from build123d import *

# Parameters (mm, degrees)
F0_W           = 101.6
F0_H           = 50.8
F1_DEPTH       = 50.8
F3_D           = 12.7
F3_CBORE_D     = 25.4
F3_CBORE_DEPTH = 6.35
F5_R           = 12.7
F6_DEPTH       = 25.4
F7_R           = 5.08


with BuildPart() as f1:
    # F0 (on Top) → F1 (new body)
    with BuildSketch(Plane.XY):
        with Locations((50.8, 25.4)):
            Rectangle(F0_W, F0_H)
    extrude(amount=F1_DEPTH)

    # F3 (through all)
    with Locations(Plane(origin=(0, 50.8, 0), x_dir=(-1, 0, 0), z_dir=(0, 1, 0))):
        with Locations((-50.8, 25.4)):
            CounterBoreHole(F3_D / 2, F3_CBORE_D / 2, F3_CBORE_DEPTH)

    # F5 (on offset) → F6 (join, through all)
    with BuildSketch(Plane(origin=(0, 0, -25.4), x_dir=(1, 0, 0), z_dir=(0, 0, -1))):
        with Locations((50.8, -26.0627344251)):
            Circle(F5_R)
    extrude(amount=-F6_DEPTH)

    # F7
    f7_edges = [f1.edges().sort_by_distance(p)[0] for p in [
        (101.6, 0, 25.4),
        (101.6, 50.8, 25.4),
        (101.6, 25.4, 0),
        (101.6, 25.4, 50.8),
        (0, 50.8, 25.4),
        (0, 0, 25.4),
        (0, 25.4, 0),
        (0, 25.4, 50.8),
        (50.8, 0, 50.8),
        (50.8, 50.8, 50.8),
        (50.8, 0, 0),
        (57.15, 0, 25.4),
        (50.8, 50.8, 0),
    ]]
    fillet(f7_edges, radius=F7_R)


solid = f1.part
For this review, take the finished solid that the model builds, in its own axes (mm). A direction names the side the tool comes from. Give positions to 0.01 mm unless a question says otherwise; leave off trailing zeros. Order: outer loops, then holes, each group sorted by start corner. A loop starts at its lowest first (then second) coordinate and runs counter-clockwise, first axis right, second up. Notation, with made-up numbers: (-21, 76.25) - (2, 76.25) arc R10 cw to (2, 95.25) - close; hole circle Ø2 at (-36, -11.5). An arc over 180 degrees is marked (long way). Answer as a JSON object with one key per item and string values. Group by question number.
Item 1: Take a section at A-A on x = 50.8. Give the boundary of the cut face in (y, z), and give its area (3 significant figures).
Item 2: Take a section at C-C on y = 40. Give the boundary of the cut face in (x, z).
Item 3: Clearance check with a flat-ended pin moving along its axis: pin 1 Ø4 at (x, y) = (85, 43.5) entering from -Z. State where the tip first meets the part, or that it passes through.
Item 4: Take a section at D-D on z = 3. Give the boundary of the cut face in (x, y), and give its area (3 significant figures).
Item 5: Draft analysis for pull direction Z (two halves, no side actions). For faces 1 (the cylindrical face through (43.973, 47.669, 36.109)), 2 (the cylindrical face through (56.666, 24.489, 22.968)), 3 (the cylindrical face through (100.072, 25.684, 49.351)), 4 (the flat face through (50, 39, 0)), state which applies: pulls with the +Z half, pulls with the -Z half, needs draft (parallel to the pull), parting line crosses it, or undercut.
Item 6: Wall thickness on line 1 along Z through (x, y) = (50.8, 22.5); line 2 along Z through (x, y) = (68, 15); line 3 along X through (y, z) = (32, 25): over which ranges is each line inside the solid? List them lowest first.
Item 7: Machinability: for faces 5 (the flat face through (101.6, 25, 25)), 6 (the cylindrical face through (38.112, 25.504, -12.878)), which of the approach directions +Z, -Z, +X, -X, +Y, -Y give a long, thin tool a straight path to every point of the face, cutting with its end or side? Answer none if there is none.
Item 8: Take a section at B-B on z = 25.4. Give the boundary of the cut face in (x, y).
Reported:
{
 "1": {"outline": "(0, 5.08) arc R5.08 ccw to (5.08, 0) - (13.36, 0) - (13.36, -25.4) - (38.76, -25.4) - (38.76, 0) - (45.72, 0) arc R5.08 ccw to (50.8, 5.08) - (50.8, 12.7) - (44.45, 12.7) - (44.45, 19.05) - (5.08, 19.05) arc R5.08 ccw to (0, 13.97) - close; (0, 36.83) arc R5.08 ccw to (5.08, 31.75) - (44.45, 31.75) - (44.45, 38.1) - (50.8, 38.1) - (50.8, 45.72) arc R5.08 ccw to (45.72, 50.8) - (5.08, 50.8) arc R5.08 ccw to (0, 45.72) - close", "area": "2,470 mm^2"},
 "2": {"outline": "(0, 5.08) arc R5.08 ccw to (5.08, 0) - (96.52, 0) arc R5.08 ccw to (101.6, 5.08) - (101.6, 45.72) arc R5.08 ccw to (96.52, 50.8) - (5.08, 50.8) arc R5.08 ccw to (0, 45.72) - close; hole circle Ø12.7 at (50.8, 25.4)"},
 "3": {"pin 1": "z = 0"},
 "4": {"outline": "(0.45, 5.08) arc R4.63 ccw to (5.08, 0.45) - (96.52, 0.45) arc R4.63 ccw to (101.15, 5.08) - (101.15, 45.72) arc R4.63 ccw to (96.52, 50.35) - (5.08, 50.35) arc R4.63 ccw to (0.45, 45.72) - close", "area": "5,010 mm^2"},
 "5": {"face 1": "undercut", "face 2": "undercut", "face 3": "pulls with the +Z half", "face 4": "pulls with the -Z half"},
 "6": {"line 1": "-25.4 to 19.05, 31.75 to 50.8", "line 2": "0 to 50.8", "line 3": "0 to 44.46, 57.14 to 101.6"},
 "7": {"face 5": "+Z, -Z, +X, +Y, -Y", "face 6": "-Z"},
 "8": {"outline": "(0, 5.08) arc R5.08 ccw to (5.08, 0) - (39.37, 0) arc R5.08 ccw to (44.45, 5.08) - (44.45, 44.45) - (38.1, 44.45) - (38.1, 50.8) - (5.08, 50.8) arc R5.08 ccw to (0, 45.72) - close; (57.15, 5.08) arc R5.08 ccw to (62.23, 0) - (96.52, 0) arc R5.08 ccw to (101.6, 5.08) - (101.6, 45.72) arc R5.08 ccw to (96.52, 50.8) - (63.5, 50.8) - (63.5, 44.45) - (57.15, 44.45) - close"}
}
